from build123d import *

# Parameters (mm, degrees)
SKETCH2_R           = 4.5
BOSS_EXTRUDE1_DEPTH = 5


with BuildPart() as part:
    # Sketch2 → Boss-Extrude1 (new, symmetric)
    with BuildSketch(Plane(origin=(0, 0, 0), x_dir=(1, 0, 0), z_dir=(0, 1, 0))):
        Polygon((107.573593129, 150), (-107.573593129, 150), (-150, 107.573593129), (-150, -107.573593129), (-107.573593129, -150), (107.573593129, -150), (150, -107.573593129), (150, 107.573593129), align=None)
        with Locations(Location((-78, 140, 0), (0, 0, 270))):
            Circle(SKETCH2_R, mode=Mode.SUBTRACT)
        with Locations(Location((78, 140, 0), (0, 0, 90))):
            Circle(SKETCH2_R, mode=Mode.SUBTRACT)
        with Locations(Location((-140, 78, 0), (0, 0, 270))):
            Circle(SKETCH2_R, mode=Mode.SUBTRACT)
        with Locations(Location((140, 78, 0), (0, 0, 90))):
            Circle(SKETCH2_R, mode=Mode.SUBTRACT)
        with Locations(Location((-140, -78, 0), (0, 0, 270))):
            Circle(SKETCH2_R, mode=Mode.SUBTRACT)
        with Locations(Location((140, -78, 0), (0, 0, 90))):
            Circle(SKETCH2_R, mode=Mode.SUBTRACT)
        with Locations(Location((-78, -140, 0), (0, 0, 270))):
            Circle(SKETCH2_R, mode=Mode.SUBTRACT)
        with Locations(Location((78, -140, 0), (0, 0, 90))):
            Circle(SKETCH2_R, mode=Mode.SUBTRACT)
    extrude(amount=BOSS_EXTRUDE1_DEPTH, both=True)


solid = part.part
Geometry check sheet. Reference: the model listing, model coordinates, mm. Round coordinates to 2 decimals unless told otherwise and drop trailing zeros. Loops run counter-clockwise (first coordinate to the right, second up) from the corner with the lowest first, then second, coordinate; pieces in that order, holes last.
Item 1: Gauge pin test, flat ends, axial feed: pin 1 (7 mm diameter, centred on x = 140, z = 78, fed in from -Y); pin 2 (14.5 mm diameter, centred on x = -78, z = -140, fed in from -Y); pin 3 (1 mm diameter, centred on x = 118, y = -3, fed in from -Z). Record the tip position at first contact, or that the pin passes through.
Item 2: Cross-section at B-B on y = -3.5. Count the separate pieces of the cut face and the enclosed holes in it, then the cut area to 3 significant figures.
Item 3: Cross-section at D-D on z = 120.5. Record the boundary of the cut face in (x, y), then the cut area to 3 significant figures.
Item 4: Thickness scan on line 1 (X direction, y = -2.25, z = 78); line 2 (Z direction, x = 140, y = -0.75). Record the ranges inside material, lowest first.
Item 5: Cross-section at C-C on z = -78. Record the boundary of the cut face in (x, y).
Item 6: Mould release check, pull along X, two halves, no side actions. Record for faces 1 (the flat face through (150, 0, 2)), 2 (the flat face through (-150, 0, -2)), 3 (the cylindrical face through (-74.206, -0.07, 142.419)), 4 (the cylindrical face through (144.39, -0.07, -77.02)): pulls with the +X half, pulls with the -X half, needs draft (parallel to the pull), parting line crosses it, or undercut.
Item 7: Cross-section at A-A on x = -78. Record the boundary of the cut face in (y, z), then the cut area to 3 significant figures.
Answer sheet:
1. pin 1: passes through
1. pin 2: stops at y = -5
1. pin 3: stops at z = -140.07
2. separate pieces: 1
2. enclosed holes: 8
2. area: 85,900 mm2
3. outline: (-137.07, -5) - (137.07, -5) - (137.07, 5) - (-137.07, 5) - close
3. area: 2,740 mm2
4. line 1: x = -150 to -144.5, -135.5 to 135.5, 144.5 to 150
4. line 2: z = -117.57 to -82.5, -73.5 to 73.5, 82.5 to 117.57
5. outline: (-150, -5) - (-144.5, -5) - (-144.5, 5) - (-150, 5) - close; (-135.5, -5) - (135.5, -5) - (135.5, 5) - (-135.5, 5) - close; (144.5, -5) - (150, -5) - (150, 5) - (144.5, 5) - close
6. face 1: pulls with the +X half
6. face 2: pulls with the -X half
6. face 3: undercut
6. face 4: undercut
7. outline: (-5, -150) - (5, -150) - (5, -144.5) - (-5, -144.5) - close; (-5, -135.5) - (5, -135.5) - (5, 135.5) - (-5, 135.5) - close; (-5, 144.5) - (5, 144.5) - (5, 150) - (-5, 150) - close
7. area: 2,820 mm2
